Autodesk Inventor part; units mm, degrees
ref_plane "YZ Plane" through (0, 0, 0) normal (1, 0, 0) x (0, 1, 0)
ref_plane "XZ Plane" through (0, 0, 0) normal (0, 1, 0) x (-1, 0, 0)
ref_plane "XY Plane" through (0, 0, 0) normal (0, 0, 1) x (1, 0, 0)
sketch "Sketch1" plane through (0, 0, 0) normal (1, 0, 0) x (0, 1, 0)
  circle A0 centre (0, 0) radius 15.95
  dimension "d0" = 31.9
extrude "Extrusion1" add sketch "Sketch1" along normal blind 8
sketch "Sketch2" plane through (8, 0, 0) normal (1, 0, 0) x (0, 0, -1)
  line L0 (-28, -20) -> (28, -20)
  line L1 (28, -20) -> (28, 40)
  line L2 (28, 40) -> (-28, 40)
  line L3 (-28, 40) -> (-28, -20)
  line L4 (-28, -20) -> (28, 40) construction
  line L5 (28, -20) -> (-28, 40) construction
  point P0 (0, 0)
  point P1 (0, 10)
  point P2 (0, 10)
  dimension "d3" = 60
  dimension "d4" = 56
  dimension "d46" = 10
extrude "Extrusion2" add sketch "Sketch2" along normal blind 42
sketch "Sketch3" plane through (8, 40, 28) normal (0, 1, 0) x (1, 0, 0)
  line L0 (0, 56) -> (42, 56)
  line L1 (21, 56) -> (21, 0) construction
  line L2 (0, 0) -> (42, 0)
  line L3 (10.5, 7.5) -> (31.5, 7.5)
  line L4 (31.5, 7.5) -> (31.5, 48.5)
  line L5 (31.5, 48.5) -> (10.5, 48.5)
  line L6 (10.5, 48.5) -> (10.5, 7.5)
  line L7 (10.5, 7.5) -> (31.5, 48.5) construction
  line L8 (31.5, 7.5) -> (10.5, 48.5) construction
  point P0 (-8, 28)
  point P1 (21, 28)
  dimension "d7" = 21
  dimension "d8" = 41
extrude "Extrusion3" cut sketch "Sketch3" against normal through all
sketch "Sketch4" plane through (50, 0, 0) normal (1, 0, 0) x (0, 0, -1)
  circle A0 centre (0, 0) radius 15.95
extrude "Extrusion4" cut sketch "Sketch4" against normal up to surface (10.5 mm away)
sketch "Sketch5" plane through (18.5, 40, 20.5) normal (1, 0, 0) x (0, 0, -1)
  circle A0 centre (20.5, -40) radius 15.95 construction
  circle A1 centre (12.5, -32) radius 2.1
  circle A2 centre (12.5, -48) radius 2.1
  circle A3 centre (28.5, -48) radius 2.1
  circle A4 centre (28.5, -32) radius 2.1
  dimension "d13" = 4.2
  dimension "d14" = 8
  dimension "d15" = 8
  dimension "d18" = 360
extrude "Extrusion5" cut sketch "Sketch5" against normal through all
sketch "Sketch6" plane through (8, 40, 28) normal (0, 1, 0) x (1, 0, 0)
  line L0 (31.5, 48.5) -> (10.5, 48.5) construction
  line L1 (21, 48.5) -> (21, 7.5) construction
  line L2 (10.5, 7.5) -> (31.5, 7.5) construction
  line L3 (0, 0) -> (42, 0)
  line L4 (0, 0) -> (42, 0)
  line L5 (42, 0) -> (42, -12)
  line L6 (42, -12) -> (0, -12)
  line L7 (0, -12) -> (0, 0)
  line L8 (10.5, 7.5) -> (10.5, 48.5) construction
  line L9 (10.5, 28) -> (31.5, 28) construction
  line L10 (31.5, 12.05) -> (31.5, 43.95) construction
  line L11 (0, 56) -> (42, 56)
  line L12 (0, 56) -> (42, 56)
  line L13 (42, 56) -> (42, 68)
  line L14 (42, 68) -> (0, 68)
  line L15 (0, 68) -> (0, 56)
  point P0 (-8, 28)
  point P1 (21, 28)
  dimension "d25" = 12
extrude "Extrusion6" add sketch "Sketch6" against normal blind 12
sketch "Sketch8" plane through (8, 40, 40) normal (0, 1, 0) x (1, 0, 0)
  line L0 (10.5, 19.5) -> (31.5, 19.5) construction
  line L1 (21, 19.5) -> (21, 60.5) construction
  line L2 (31.5, 60.5) -> (10.5, 60.5) construction
  circle A0 centre (26, 16) radius 2.1
  line L3 (31.5, 19.5) -> (10.5, 19.5)
  line L4 (10.5, 19.5) -> (10.5, 60.5) construction
  line L5 (10.5, 40) -> (31.5, 40) construction
  line L6 (31.5, 24.05) -> (31.5, 55.95) construction
  circle A1 centre (16, 16) radius 2.1
  circle A2 centre (26, 64) radius 2.1
  circle A3 centre (16, 64) radius 2.1
  point P0 (-8, 40)
  point P1 (21, 40)
  dimension "d31" = 4.2
  dimension "d32" = 5
  dimension "d33" = 24
extrude "Extrusion8" cut sketch "Sketch8" against normal up to surface (12 mm away)
fillet "Fillet2" radius 4 2 edges at (50, 34, 40) (50, 34, -40)
chamfer "Chamfer1" distance 2 angle 45 1 edges at (50, 0, 15.95)
chamfer "Chamfer2" distance 8 angle 45 2 edges at (29, 28, 28) (29, 28, -28)
sketch "Sketch10" plane through (8, 40, 40) normal (0, 1, 0) x (1, 0, 0)
  line L0 (31.5, 60.5) -> (10.5, 60.5) construction
  line L1 (21, 60.5) -> (21, 19.5) construction
  line L2 (31.5, 19.5) -> (10.5, 19.5) construction
  circle A0 centre (5, 33.97) radius 2.1
  circle A1 centre (5, 65.97) radius 2.1
  circle A2 centre (37, 33.97) radius 2.1
  circle A3 centre (37, 65.97) radius 2.1
  line L3 (0, 80) -> (0, 0) construction
  line L4 (0, 73.97) -> (10.5, 73.97)
  line L5 (10.5, 73.97) -> (10.5, 25.97)
  line L6 (10.5, 25.97) -> (0, 25.97)
  line L7 (0, 25.97) -> (0, 73.97)
  line L8 (5, 65.97) -> (5, 33.97) construction
  line L9 (42, 73.97) -> (31.5, 73.97)
  line L10 (31.5, 73.97) -> (31.5, 25.97)
  line L11 (31.5, 25.97) -> (42, 25.97)
  line L12 (42, 25.97) -> (42, 73.97)
  point P0 (-8, 40)
  point P1 (21, 40)
  point P2 (10.5, 49.97)
  point P3 (5, 49.97)
  dimension "d58" = 4.2
  dimension "d60" = 16
  dimension "d61" = 4.2
  dimension "d62" = 32
  dimension "d63" = 48
  dimension "d64" = 10.5
  dimension "d67" = 9.97
extrude "Extrusion10" add sketch "Sketch10" along normal blind 14.8
properties part number "VerticalAxisServoMount"
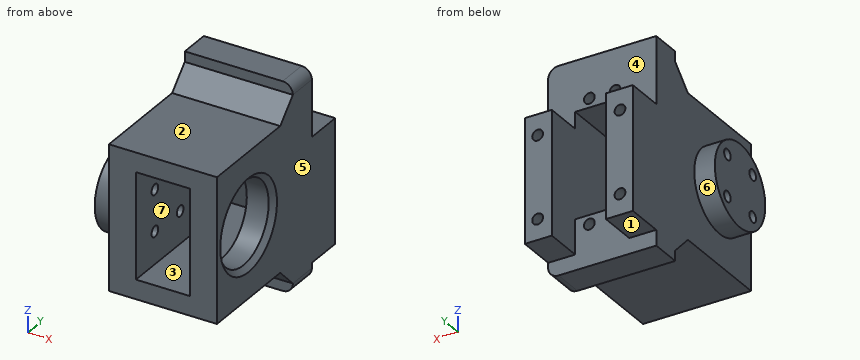
Design review of the part built by this model. Coordinates are the model's own, in mm. Face numbers are marked on the shaded views. A direction names the side the tool comes from. Coordinates: 2 decimals unless noted, no trailing zeros. Order: outer loops, then holes, each group sorted by start corner. A loop starts at its lowest first (then second) coordinate and runs counter-clockwise, first axis right, second up. Notation, with made-up numbers: (28.25, -8.75) - (57.25, -8.75) arc R7 ccw to (57.25, 2.25) - close; hole circle Ø7 at (-4.5, 82). An arc over 180 degrees is marked (long way). Answer in a Markdown table with one row per item.
(1) Consider section C-C on z = -32. State the section outline as (x, y) points, plus the area to 3 significant figures.
Checked values:
| item | result |
|---|---|
| outline | (8, 24) - (50, 24) - (50, 54.8) - (39.5, 54.8) - (39.5, 40) - (18.5, 40) - (18.5, 54.8) - (8, 54.8) - close |
| area | 983 mm^2 |
(2) Consider section B-B on x = 45. State the section outline as (y, z) points, plus the area to 3 significant figures.
Checked values:
| item | result |
|---|---|
| outline | (-20, -28) - (20, -28) - (28, -36) - (28, -40) - (40, -40) - (40, -33.97) - (54.8, -33.97) - (54.8, -28.07) - (40, -28.07) - (40, -23.87) - (54.8, -23.87) - (54.8, 3.93) - (40, 3.93) - (40, 8.13) - (54.8, 8.13) - (54.8, 14.03) - (40, 14.03) - (40, 40) - (28, 40) - (28, 36) - (20, 28) - (-20, 28) - close; hole circle Ø31.9 at (0, 0) |
| area | 3,500 mm^2 |
(3) Consider section A-A on y = 45. State the section outline as (x, z) points, plus the area to 3 significant figures.
Checked values:
| item | result |
|---|---|
| outline | (8, -33.97) - (18.5, -33.97) - (18.5, 14.03) - (8, 14.03) - close; (39.5, -33.97) - (50, -33.97) - (50, 14.03) - (39.5, 14.03) - close; hole circle Ø4.2 at (13, -25.97); hole circle Ø4.2 at (13, 6.03); hole circle Ø4.2 at (45, -25.97); hole circle Ø4.2 at (45, 6.03) |
| area | 953 mm^2 |
(4) Consider section D-D on x = 34. State the section outline as (y, z) points, plus the area to 3 significant figures.
Checked values:
| item | result |
|---|---|
| outline | (-20, -28) - (20, -28) - (28, -36) - (28, -40) - (40, -40) - (40, -26.1) - (28, -26.1) - (28, -21.9) - (40, -21.9) - (40, -20.5) - (-20, -20.5) - close; (-20, 20.5) - (40, 20.5) - (40, 21.9) - (28, 21.9) - (28, 26.1) - (40, 26.1) - (40, 40) - (28, 40) - (28, 36) - (20, 28) - (-20, 28) - close |
| area | 1,150 mm^2 |
(5) Clearance check with flat-ended pins moving along their axes: pin 1 (4.5 mm diameter, centred on x = 34.5, z = 23, fed in from +Y); pin 2 (8.5 mm diameter, centred on x = 47, y = 48.5, fed in from -Z); pin 3 (5 mm diameter, centred on y = 8, z = -8, fed in from +X). State where each tip first meets the part, or that it passes through.
Checked values:
| item | result |
|---|---|
| pin 1 | y = 40 |
| pin 2 | z = -33.97 |
| pin 3 | x = 18.5 |
(6) Wall thickness on line 1 along Z through (x, y) = (24, 30.5); line 2 along Y through (x, z) = (11.25, 8); line 3 along Y through (x, z) = (13, 8): over which ranges is each line inside the solid? List them lowest first. Write a range as from..to.
Checked values:
| item | result |
|---|---|
| line 1 | -40..-26.1, -21.9..-20.5, 20.5..21.9, 26.1..40 |
| line 2 | -20..-10.1, -5.9..5.9, 10.1..54.8 |
| line 3 | -20..-10.1, -5.9..5.9, 10.1..40 |
(7) For the marked faces 1, 2, 3 and 4, list the 3-axis set-ups (+Z, -Z, +X, -X, +Y, -Y) from which the entire face can be reached by the end or side of a thin tool; tool diameter is ignored.
Checked values:
| item | result |
|---|---|
| face 1 | -Z, +X, -X, +Y |
| face 2 | +Z, +X, -X, -Y |
| face 3 | +Y, -Y |
| face 4 | +Z, +X, -X, +Y |
(8) The part is to be moulded in two halves that separate along X. For the marked faces 5, 6 and 7, say which applies: released by +X, released by -X, zero draft, split by the parting line, or undercut.
Checked values:
| item | result |
|---|---|
| face 5 | released by +X |
| face 6 | zero draft |
| face 7 | undercut |
